from build123d import *

# Parameters (mm, degrees)
ESQUISSE1_W             = 424
ESQUISSE1_H             = 460
BOSS_EXTRU_1_DEPTH      = 10
ENL_V_MAT_EXTRU_1_DEPTH = 5
CHANFREIN1_SIZE         = 5


with BuildPart() as part:
    # Esquisse1 → Boss.-Extru.1 (new body)
    with BuildSketch(Plane.XY):
        with Locations((212, 230)):
            Rectangle(ESQUISSE1_W, ESQUISSE1_H)
    extrude(amount=BOSS_EXTRU_1_DEPTH)

    # Esquisse2 → Enlèv. mat.-Extru.1 (cut)
    with BuildSketch(Plane.XY.offset(10)):
        Polygon((95, 226.923881554), (95, 233.076118446), (40, 288.076118446), (40, 171.923881554), align=None)
        Polygon((191.923881554, 320), (232.076118446, 320), (332.076118446, 420), (91.923881554, 420), align=None)
        Polygon((40, 420), (40, 330.502525317), (130, 240.502525317), (130, 219.497474683), (40, 129.497474683), (40, 40), (49.497474683, 40), (179.497474683, 170), (244.502525317, 170), (374.502525317, 40), (384, 40), (384, 129.497474683), (294, 219.497474683), (294, 240.502525317), (384, 330.502525317), (384, 420), (374.502525317, 420), (244.502525317, 290), (179.497474683, 290), (49.497474683, 420), align=None)
        Polygon((329, 226.923881554), (329, 233.076118446), (384, 288.076118446), (384, 171.923881554), align=None)
        Polygon((332.076118446, 40), (91.923881554, 40), (191.923881554, 140), (232.076118446, 140), align=None)
    extrude(amount=-ENL_V_MAT_EXTRU_1_DEPTH, mode=Mode.SUBTRACT)

    # Chanfrein1
    chanfrein1_edges = [part.edges().sort_by_distance(p)[0] for p in [
        (212, 40, 5),
        (141.923881554, 90, 5),
        (212, 140, 5),
        (282.076118446, 90, 5),
        (40, 230, 5),
        (67.5, 260.576118446, 5),
        (95, 230, 5),
        (67.5, 199.423881554, 5),
        (384, 230, 5),
        (356.5, 199.423881554, 5),
        (329, 230, 5),
        (356.5, 260.576118446, 5),
        (114.497474683, 355, 5),
        (212, 290, 5),
        (309.502525317, 355, 5),
        (379.251262658, 420, 5),
        (384, 375.251262658, 5),
        (339, 285.502525317, 5),
        (294, 230, 5),
        (339, 174.497474683, 5),
        (384, 84.748737342, 5),
        (379.251262658, 40, 5),
        (309.502525317, 105, 5),
        (212, 170, 5),
        (114.497474683, 105, 5),
        (44.748737342, 40, 5),
        (40, 84.748737342, 5),
        (85, 174.497474683, 5),
        (130, 230, 5),
        (85, 285.502525317, 5),
        (40, 375.251262658, 5),
        (44.748737342, 420, 5),
        (212, 420, 5),
        (282.076118446, 370, 5),
        (212, 320, 5),
        (141.923881554, 370, 5),
    ]]
    chamfer(chanfrein1_edges, length=CHANFREIN1_SIZE - 0.0001)  # a hair under: the kernel refuses the full size


solid = part.part
The model under review builds one solid part; all positions refer to its coordinate system, in mm. A direction names the side the tool comes from. Give positions to 0.01 mm unless a question says otherwise; leave off trailing zeros.
1. Add section B-B, the plane z = 7. Count the separate pieces of the cut face and the enclosed holes in it, plus the area to 3 significant figures.
2. Tool access review of faces 3 (the flat face through (358.677, 200.831, 7.465)), 4 (the flat face through (424, 227, 5)): name each direction out of +Z, -Z, +X, -X, +Y, -Y from which nothing blocks a thin tool from reaching the whole face with its end or side.
3. Draft analysis for pull direction Y (two halves, no side actions). For faces 1 (the flat face through (0, 227, 5)), 2 (the flat face through (309.643, 108.445, 7.465)), state which applies: +Y half, -Y half, draft (parallel to the pull), parting line (faces both ways), or undercut.
4. Wall thickness on L1, parallel to X at y = 84.5, z = 8.75; L2, parallel to X at y = 392, z = 8; L3, parallel to Y at x = 312, z = 7.5: over which ranges is each line inside the solid? List them lowest first.
Worked answers:
1. separate pieces: 1
1. enclosed holes: 5
1. area: 110,000 mm2
2. face 3: +Z
2. face 4: +Z, -Z, +X, +Y, -Y
3. face 1: draft
3. face 2: undercut
4. L1: x = 0 to 41.25, 92.23 to 138.19, 285.81 to 331.77, 382.75 to 424
4. L2: x = 0 to 42, 74.67 to 122.75, 301.25 to 349.33, 382 to 424
4. L3: y = 0 to 42.5, 56.54 to 106.04, 197.96 to 262.04, 353.96 to 403.46, 417.5 to 460
